```python
from build123d import *

# Parameters (mm, degrees)
SKETCH3_R             = 1.6
BOSS_EXTRUDE1_DEPTH   = 27.4
BOSS_EXTRUDE1_2_DEPTH = 27.4
BOSS_EXTRUDE1_3_DEPTH = 27.4
BOSS_EXTRUDE1_4_DEPTH = 27.4
SKETCH3_R_2           = 3.975
BOSS_EXTRUDE1_5_DEPTH = 27.4
SKETCH3_17_R          = 10.9
BOSS_EXTRUDE2_DEPTH   = 2


with BuildPart() as part:
    # Sketch3 → Boss-Extrude1 (new body)
    with BuildSketch(Plane(origin=(0, 0, 0), x_dir=(1, 0, 0), z_dir=(0, 1, 0))):
        with Locations(Location((0.009034474, 8.115584077, 0), (0, 0, 90))):
            Circle(SKETCH3_R)
    extrude(amount=BOSS_EXTRUDE1_DEPTH)



with BuildPart() as body_2:
    # Sketch3 → Boss-Extrude1 2 (new body)
    with BuildSketch(Plane(origin=(0, 0, 0), x_dir=(1, 0, 0), z_dir=(0, 1, 0))):
        with Locations(Location((8.017679827, 0.053335715, 0), (0, 0, 90))):
            Circle(SKETCH3_R)
    extrude(amount=BOSS_EXTRUDE1_2_DEPTH)


with BuildPart() as body_3:
    # Sketch3 → Boss-Extrude1 3 (new body)
    with BuildSketch(Plane(origin=(0, 0, 0), x_dir=(1, 0, 0), z_dir=(0, 1, 0))):
        with Locations(Location((0.009179949, -8.009057152, 0), (0, 0, 90))):
            Circle(SKETCH3_R)
    extrude(amount=BOSS_EXTRUDE1_3_DEPTH)


with BuildPart() as body_4:
    # Sketch3 → Boss-Extrude1 4 (new body)
    with BuildSketch(Plane(origin=(0, 0, 0), x_dir=(1, 0, 0), z_dir=(0, 1, 0))):
        with Locations(Location((-7.999465404, 0.05319121, 0), (0, 0, 90))):
            Circle(SKETCH3_R)
    extrude(amount=BOSS_EXTRUDE1_4_DEPTH)


with BuildPart() as body_5:
    # Sketch3 → Boss-Extrude1 5 (new body)
    with BuildSketch(Plane(origin=(0, 0, 0), x_dir=(1, 0, 0), z_dir=(0, 1, 0))):
        with Locations(Location((0, 0, 0), (0, 0, 90))):
            Circle(SKETCH3_R_2)
        with BuildLine():
            Line((-1.823098343, 2.445161023), (1.823098343, 2.445161023))
            ThreePointArc((1.823098343, 2.445161023), (0, -3.05), (-1.823098343, 2.445161023))
        make_face(mode=Mode.SUBTRACT)
    extrude(amount=BOSS_EXTRUDE1_5_DEPTH)


with BuildPart() as part_1:
    add(part.part)

    add(body_2.part)  # Boss-Extrude2 merges body 2

    add(body_3.part)  # Boss-Extrude2 merges body 3

    add(body_4.part)  # Boss-Extrude2 merges body 4

    add(body_5.part)  # Boss-Extrude2 merges body 5
    # Sketch3_17 → Boss-Extrude2 (add)
    with BuildSketch(Plane(origin=(0, 0, 0), x_dir=(1, 0, 0), z_dir=(0, 1, 0))):
        with Locations(Location((0, 0, 0), (0, 0, 270))):
            Circle(SKETCH3_17_R)
    extrude(amount=BOSS_EXTRUDE2_DEPTH)


solid = part_1.part
```
Build history of the part. All positions in model axes, mm. A direction names the side the tool comes from. Round coordinates to 2 decimals unless told otherwise and drop trailing zeros. Order: outer loops, then holes, each group sorted by start corner. A loop starts at its lowest first (then second) coordinate and runs counter-clockwise, first axis right, second up. Notation, with made-up numbers: (-34, -22.5) - (14, -22.5) arc R25 cw to (14, 9.5) - close; hole circle Ø3 at (32.25, 1). An arc over 180 degrees is marked (long way). Use a Markdown table: item, result.
1) Flat gauge pins, fed straight in: pin 1 Ø6 at (y, z) = (15, 5.5) entering from +X; pin 2 Ø1.5 at (x, y) = (3, 10) entering from -Z; pin 3 Ø12 at (y, z) = (10, 5) entering from +X. Where does each tip first touch, or does it go through?
Recorded:
| item | result |
|---|---|
| pin 1 | stops at x = 3.09 |
| pin 2 | stops at z = -3.28 |
| pin 3 | stops at x = 9.62 |
2) Tool access for faces 5 (the face through (0, 2, 5)), 6 (the face through (0, 27.4, -3)): list every direction of +Z, -Z, +X, -X, +Y, -Y with a clear straight run to the whole face (end or side of a thin tool).
Recorded:
| item | result |
|---|---|
| face 5 | +Y |
| face 6 | +Z, -Z, +X, -X, +Y |
3) Saw through at A-A on y = 9.5. Write the cut outline in (x, z) (3 decimals), and give its area (3 significant figures).
Recorded:
| item | result |
|---|---|
| outline | circle Ø3.2 at (-7.999, -0.053); circle Ø7.95 at (0, 0); circle Ø3.2 at (0.009, -8.116); circle Ø3.2 at (0.009, 8.009); circle Ø3.2 at (8.018, -0.053); hole (-1.823, -2.445) - (1.823, -2.445) arc R3.05 ccw (long way) to start |
| area | 54.1 mm² |
4) Pull direction X, two halves, no side cores. Call faces 1 (the face through (-0.061, 14.522, 9.608)), 2 (the face through (0, 2, 0)), 3 (the face through (0, 0, 0)), 4 (the face through (-9.35, 14.52, -0.91)): pulls with the +X half, pulls with the -X half, needs draft (parallel to the pull), parting line crosses it, or undercut.
Recorded:
| item | result |
|---|---|
| face 1 | parting line crosses it |
| face 2 | undercut |
| face 3 | needs draft |
| face 4 | undercut |
5) Saw through at B-B on x = -1.25. Write the cut outline in (y, z), and give its area (3 significant figures).
Recorded:
| item | result |
|---|---|
| outline | (0, -10.83) - (2, -10.83) - (2, -9.1) - (27.4, -9.1) - (27.4, -7.13) - (2, -7.13) - (2, -3.77) - (27.4, -3.77) - (27.4, -2.45) - (2, -2.45) - (2, 2.78) - (27.4, 2.78) - (27.4, 3.77) - (2, 3.77) - (2, 7.02) - (27.4, 7.02) - (27.4, 9) - (2, 9) - (2, 10.83) - (0, 10.83) - close |
| area | 203 mm² |
6) Wall check: L1, parallel to X at y = 20.5, z = 0 (3 decimals); L2, parallel to Y at x = 6.25, z = -5.5; L3, parallel to X at y = 18, z = 1. Give the ranges that are in metal, low to high.
Recorded:
| item | result |
|---|---|
| L1 | x = -9.599 to -6.4, -3.975 to -3.05, 3.05 to 3.975, 6.419 to 9.617 |
| L2 | y = 0 to 2 |
| L3 | x = -9.2 to -6.79, -3.85 to -2.88, 2.88 to 3.85, 6.81 to 9.22 |
7) Saw through at D-D on z = -6. Write the cut outline in (x, y).
Recorded:
| item | result |
|---|---|
| outline | (-9.1, 0) - (9.1, 0) - (9.1, 2) - (-9.1, 2) - close |
8) Saw through at C-C on z = 0. Write the cut outline in (x, y) (3 decimals).
Recorded:
| item | result |
|---|---|
| outline | (-10.9, 0) - (10.9, 0) - (10.9, 2) - (9.617, 2) - (9.617, 27.4) - (6.419, 27.4) - (6.419, 2) - (3.975, 2) - (3.975, 27.4) - (3.05, 27.4) - (3.05, 2) - (-3.05, 2) - (-3.05, 27.4) - (-3.975, 27.4) - (-3.975, 2) - (-6.4, 2) - (-6.4, 27.4) - (-9.599, 27.4) - (-9.599, 2) - (-10.9, 2) - close |
